Job drawing, mm, ordinate dimensions from the low corner. One solid piece. Give positions to 0.01 mm unless a question says otherwise; leave off trailing zeros. Loops run counter-clockwise (first coordinate to the right, second up) from the corner with the lowest first, then second, coordinate; pieces in that order, holes last. Notation, with made-up numbers: (67.25, 11.25) -> (106.25, 11.25) arc R27 ccw to (106.25, 33.25) -> close; hole circle Ø10 at (7, 75.25). An arc over 180 degrees is marked (long way). Answer as a JSON object with one key per item and string values. Group by question number.
Q1. Band-saw the part on A-A, the plane z = 5.5. Write the cut outline in (x, y), plus the area to 3 significant figures.
Q2. Wall check: probe 1 along X at (y, z) = (237, 6.5). Give the ranges that are in metal, low to high. Write a range as from..to.
Q3. Drop a flat-ended pin along its axis: pin 1 (12.5 mm diameter, centred on y = 175.5, z = 6.5, fed in from -X). Give the stop position or say it passes through.
Q4. Band-saw the part on B-B, the plane x = 215. Write the cut outline in (y, z).
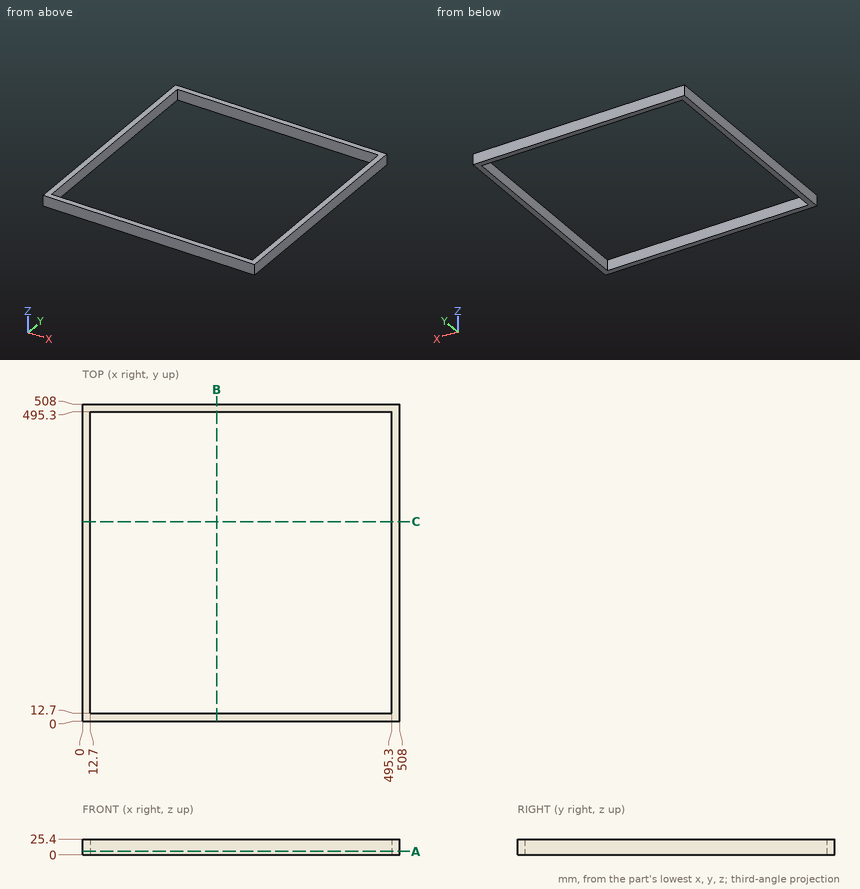
Worked answers:
{
 "1": {"outline": "(0, 0) -> (508, 0) -> (508, 508) -> (0, 508) -> close; hole (12.7, 12.7) -> (495.3, 12.7) -> (495.3, 495.3) -> (12.7, 495.3) -> close", "area": "25,200 mm2"},
 "2": {"probe 1": "0..12.7, 495.3..508"},
 "3": {"pin 1": "x = 0"},
 "4": {"outline": "(0, 0) -> (12.7, 0) -> (12.7, 25.4) -> (0, 25.4) -> close; (495.3, 0) -> (508, 0) -> (508, 25.4) -> (495.3, 25.4) -> close"}
}
